Input: part model. Units: mm. Frame: model coordinates. A direction names the side the tool comes from. Round coordinates to 2 decimals unless told otherwise and drop trailing zeros. Loops run counter-clockwise (first coordinate to the right, second up) from the corner with the lowest first, then second, coordinate; pieces in that order, holes last.
(1) Cut plane B-B, the plane y = 13.5. Output: boundary loops of the cut face in (x, z), and give its area (3 significant figures).
(2) Line query: line 1 (X direction, y = 9.25, z = -3.5); line 2 (X direction, y = 14.5, z = 16); line 3 (Y direction, x = -6, z = 10.5). Output: solid intervals per line, ascending.
(3) First-contact query: pin 1 Ø5 at (y, z) = (13.5, 16.5) entering from -X; pin 2 Ø10 at (y, z) = (10.5, 0.5) entering from +X; pin 3 Ø10 at (x, y) = (3, 9.5) entering from -Z. Flat tips, straight axial feed; report the tip coordinate or a pass-through.
(4) Draft query along Y for faces 1 (the face through (2.121, 20.763, -0.813)), 2 (the face through (-7, 1.714, 0)), 3 (the face through (2, 14, 23.948)), 4 (the face through (2, 9, 5.448)). Return one class per face: released by +Y, released by -Y, zero draft, split by the parting line, or undercut.
(5) Cut plane D-D, the plane z = 21. Output: boundary loops of the cut face in (x, y), and give its area (3 significant figures).
(6) Access query for faces 5 (the face through (2.7, 15.73, 20.45)), 6 (the face through (8.331, 8, -1)), 7 (the face through (2, 11, -7.252)), 8 (the face through (2.424, 11.043, 12.992)). Directions: +Z, -Z, +X, -X, +Y, -Y. A direction counts if a zero-diameter tool reaches every point of the face in a straight line with its end or side. Return the directions, or none.
(7) Cut plane C-C, the plane x = -3.5. Output: boundary loops of the cut face in (y, z), and give its area (3 significant figures).
(8) Cut plane A-A, the plane z = 6. Output: boundary loops of the cut face in (x, y).
from build123d import *

# Parameters (mm, degrees)
SKETCH1_W           = 19.304
SKETCH1_H           = 22.225
BOSS_EXTRUDE1_DEPTH = 1.7145
SKETCH2_W           = 12.7
SKETCH2_H           = 12.7
BOSS_EXTRUDE2_DEPTH = 19.05
FILLET1_RADIUS      = 6.35
FILLET1_LENGTH      = 12.7
CUT_EXTRUDE1_START  = -6.9
CUT_EXTRUDE1_DEPTH  = 6.9


with BuildPart() as part:
    # Sketch1 → Boss-Extrude1 (new body)
    with BuildSketch(Plane(origin=(0, 0, 0), x_dir=(1, 0, 0), z_dir=(0, 1, 0))):
        Rectangle(SKETCH1_W, SKETCH1_H)
    extrude(amount=BOSS_EXTRUDE1_DEPTH)

    # Sketch2 → Boss-Extrude2 (add)
    with BuildSketch(Plane(origin=(0, 1.7145, 0), x_dir=(1, 0, 0), z_dir=(0, 1, 0))):
        with Locations((1.9812, 0.9017)):
            Rectangle(SKETCH2_W, SKETCH2_H)
    extrude(amount=BOSS_EXTRUDE2_DEPTH)

    # Fillet1: full round fillet: the end face becomes a half cylinder, R = half its width
    fillet1_face = Plane((1.9812, 20.7645, -0.9017), x_dir=(0, 0, 1), z_dir=(0, 1, 0))  # on the end face: x along it, z out of the body
    fillet1_slab = fillet1_face.offset(-FILLET1_RADIUS / 2) * Box(FILLET1_LENGTH, 2 * FILLET1_RADIUS, FILLET1_RADIUS, mode=Mode.PRIVATE)  # the body's end, R deep
    fillet1_round = Plane((1.9812, 14.4145, -0.9017), x_dir=(0, 1, 0), z_dir=(0, 0, 1)) * Cylinder(FILLET1_RADIUS, FILLET1_LENGTH, mode=Mode.PRIVATE)  # its axis R under the face
    add(fillet1_slab - fillet1_round, mode=Mode.SUBTRACT)

    # Sketch6 → Revolve1 (revolve)
    with BuildSketch(Plane(origin=(0, 14.4145, 0), x_dir=(1, 0, 0), z_dir=(0, 1, 0))):
        Polygon((1.9812, -23.9483), (-1.0188, -23.9483), (-1.0188, -17.0483), (-1.4188, -17.0483), (-1.4188, -9.0483), (-2.3588, -9.0483), (-2.3588, -5.4483), (1.9812, -5.4483), align=None)
    revolve(axis=Axis((1.9812, 14.4145, 5.4483), (0, 0, 1)))

    # Sketch7 → Cut-Extrude1 (cut)
    with BuildSketch(Plane.XY.offset(23.9483).offset(CUT_EXTRUDE1_START)):
        with BuildLine():
            Line((0.4812, 17.012576211), (4.9812, 14.4145))
            ThreePointArc((4.9812, 14.4145), (3.4812, 17.012576211), (0.4812, 17.012576211))
        make_face()
    extrude(amount=CUT_EXTRUDE1_DEPTH, mode=Mode.SUBTRACT)


solid = part.part
Reported:
1. outline: (-4.37, -7.25) - (8.33, -7.25) - (8.33, 5.45) - (6.22, 5.45) - (6.22, 9.05) - (5.26, 9.05) - (5.26, 17.05) - (4.84, 17.05) - (4.84, 23.95) - (-0.88, 23.95) - (-0.88, 17.05) - (-1.29, 17.05) - (-1.29, 9.05) - (-2.26, 9.05) - (-2.26, 5.45) - (-4.37, 5.45) - close
1. area: 284 mm2
2. line 1: x = -4.37 to 8.33
2. line 2: x = -1.42 to 5.38
2. line 3: y = 0 to 1.71
3. pin 1: stops at x = -1.42
3. pin 2: stops at x = 8.33
3. pin 3: stops at z = -7.25
4. face 1: released by +Y
4. face 2: undercut
4. face 3: zero draft
4. face 4: undercut
5. outline: (0.48, 17.01) arc R3 ccw (long way) to (4.98, 14.41) - close
5. area: 22.7 mm2
6. face 5: +Z, +X, +Y
6. face 6: +Z, -Z, +X, +Y
6. face 7: -Z, +X, -X, +Y
6. face 8: +Z
7. outline: (0, -11.11) - (1.71, -11.11) - (1.71, -7.25) - (17.62, -7.25) - (17.62, 5.45) - (1.71, 5.45) - (1.71, 11.11) - (0, 11.11) - close
7. area: 240 mm2
8. outline: (-9.65, 0) - (9.65, 0) - (9.65, 1.71) - (-9.65, 1.71) - close; circle Ø8.68 at (1.98, 14.41)
